```python
from build123d import *

# Parameters (mm, degrees)
SKETCH1_R               = 2
BOSS_EXTRUDE1_DEPTH     = 35
SKETCH2_R               = 2
BOSS_EXTRUDE2_DEPTH     = 5
SKETCH3_R               = 1
FILLET1_R               = 0.5
SKETCH4_R               = 0.55
CUT_EXTRUDE1_DEPTH      = 30.858564979
CUT_EXTRUDE1_DEPTH_BACK = 1


with BuildPart() as part:
    # Sketch1 → Boss-Extrude1 (new body)
    with BuildSketch(Plane.XY):
        with Locations((27.858564979, 100.826239149)):
            Circle(SKETCH1_R)
    extrude(amount=-BOSS_EXTRUDE1_DEPTH)

    # Sketch2 → Boss-Extrude2 (add)
    with BuildSketch(Plane.XY):
        with Locations((27.858564979, 100.826239149)):
            Circle(SKETCH2_R)
    extrude(amount=BOSS_EXTRUDE2_DEPTH)

    # Sketch3 → Cut-Revolve1 (revolve, cut)
    with BuildSketch(Plane(origin=(27.858564979, 0, 0), x_dir=(0, 0, -1), z_dir=(1, 0, 0))):
        with Locations((-2.5, 103.326239149)):
            Circle(SKETCH3_R)
    revolve(axis=Axis((27.858564979, 100.826239149, -35), (0, 0, 1)), mode=Mode.SUBTRACT)

    # Fillet1
    fillet1_edges = [part.edges().sort_by_distance(p)[0] for p in [
        (25.858564979, 100.826239149, -35),
        (25.858564979, 100.826239149, 5),
    ]]
    fillet(fillet1_edges, radius=FILLET1_R)

    # Sketch4 → Cut-Extrude1 (cut, two sides)
    with BuildSketch(Plane(origin=(0, 0, 0), x_dir=(0, 0, -1), z_dir=(1, 0, 0))) as cut_extrude1_sk:
        with Locations((32.5, 100.826239149)):
            Circle(SKETCH4_R)
        with Locations((8.5, 100.826239149)):
            Circle(SKETCH4_R)
    extrude(amount=CUT_EXTRUDE1_DEPTH, mode=Mode.SUBTRACT)
    extrude(cut_extrude1_sk.sketch, amount=-CUT_EXTRUDE1_DEPTH_BACK, mode=Mode.SUBTRACT)


solid = part.part
```
Here's how the part is built. I have some questions about the finished solid (model axes, mm). Round coordinates to 2 decimals unless told otherwise and drop trailing zeros. Loops run counter-clockwise (first coordinate to the right, second up) from the corner with the lowest first, then second, coordinate; pieces in that order, holes last. Notation, with made-up numbers: (7, -31.5) -> (29, -31.5) arc R11 cw to (29, -24.5) -> close; hole circle Ø11 at (60.5, 13). An arc over 180 degrees is marked (long way). Answer as CSV lines item,"result". Start each with the question number.
1. I need wall thicknesses on probe 1 along Y at (x, z) = (28, -32.5); probe 2 along Z at (x, y) = (26.65, 100.55); probe 3 along Y at (x, z) = (27.75, 1.5). Which ranges of each line are inside material? Lowest first, please. Write a range as from..to.
2. Imagine slicing it at B-B on x = 27.15. State how many separate pieces and enclosed holes the cut face has, plus the area to 3 significant figures.
3. If we mould it in two halves opening along Z, with no side actions, what happens to faces 1 (the face through (27.83, 100.29, -8.38)), 2 (the face through (28, 101, 5)), 3 (the face through (28, 101, -35))? For each: pulls with the +Z half, pulls with the -Z half, needs draft (parallel to the pull), parting line crosses it, or undercut.
4. Imagine slicing it at C-C on z = -14. Write out the boundary of the cut face in (x, y).
5. I'm going to push a flat-ended pin straight in: P1, Ø2, axis at y = 99.5, z = -11.5, coming from the +X side. Where does the tip first touch, or does it pass through?
6. Imagine slicing it at A-A on z = -32.5. Write out the boundary of the cut face in (x, y), plus the area to 3 significant figures.
Solution:
1,probe 1,"98.83..100.28, 101.38..102.82"
1,probe 2,"-35..-32.98, -32.02..-8.98, -8.02..5"
1,probe 3,"98.83..102.82"
2,separate pieces,"1"
2,enclosed holes,"2"
2,area,"146 mm²"
3,face 1,"undercut"
3,face 2,"pulls with the +Z half"
3,face 3,"pulls with the -Z half"
4,outline,"circle Ø4 at (27.86, 100.83)"
5,P1,"x = 29.83"
6,outline,"(25.94, 100.28) arc R2 ccw to (29.78, 100.28) -> close; (25.94, 101.38) -> (29.78, 101.38) arc R2 ccw to start"
6,area,"8.22 mm²"
